from build123d import *

# Parameters (mm, degrees)
F2_W     = 10
F2_H     = 4.472136
F3_W     = 10
F3_H     = 4.472136
F4_W     = 10
F4_H     = 4.472136
F8_ANGLE = -5


with BuildPart() as f5:
    # F4 (on offset) → F5 section 0
    with BuildSketch(Plane.XZ.offset(-30)):
        Polygon((-10, 30), (-10, 34.472136), (-13.577709, 27.316718), (-21.422291, 11.627553), (-25, 4.472136), (-25, 0), align=None)
    # F3 (on Front) → F5 section 1
    with BuildSketch(Plane.XZ):
        Polygon((-10, 30), (-10, 34.472136), (-12.398913, 29.674309), (-13.577709, 27.316718), (-21.422291, 11.627553), (-22.601087, 9.269963), (-25, 4.472136), (-25, 0), align=None)
    # F2 (on offset) → F5 section 2
    with BuildSketch(Plane.XZ.offset(30)):
        Polygon((-10, 30), (-10, 34.472136), (-11.284195, 31.903745), (-12.236068, 30), (-22.763932, 8.944272), (-23.715805, 7.040526), (-25, 4.472136), (-25, 0), align=None)
    loft()

    # F2 (on offset) → F6 section 0
    with BuildSketch(Plane.XZ.offset(30)):
        with Locations((-5, 32.236068)):
            Rectangle(F2_W, F2_H)
    # F3 (on Front) → F6 section 1
    with BuildSketch(Plane.XZ):
        with Locations((-5, 32.236068)):
            Rectangle(F3_W, F3_H)
    # F4 (on offset) → F6 section 2
    with BuildSketch(Plane.XZ.offset(-30)):
        with Locations((-5, 32.236068)):
            Rectangle(F4_W, F4_H)
    loft()

    # F2 (on offset) → F7 section 0
    with BuildSketch(Plane.XZ.offset(30)):
        with Locations((-30, 2.236068)):
            Rectangle(F2_W, F2_H)
    # F3 (on Front) → F7 section 1
    with BuildSketch(Plane.XZ):
        with Locations((-30, 2.236068)):
            Rectangle(F3_W, F3_H)
    # F4 (on offset) → F7 section 2
    with BuildSketch(Plane.XZ.offset(-30)):
        with Locations((-30, 2.236068)):
            Rectangle(F4_W, F4_H)
    loft()

    # F2 (on offset) → F8 (revolve)
    with BuildSketch(Plane.XZ.offset(30)):
        Polygon((-10, 30), (-10, 34.472136), (-11.284195, 31.903745), (-12.236068, 30), (-22.763932, 8.944272), (-23.715805, 7.040526), (-25, 4.472136), (-25, 0), align=None)
        with Locations((-5, 32.236068)):
            Rectangle(F2_W, F2_H)
        with Locations((-30, 2.236068)):
            Rectangle(F2_W, F2_H)
    revolve(axis=Axis((-35, -30, 2.236068), (0, 0, 1)), revolution_arc=F8_ANGLE)


solid = f5.part
Could you check a few things on this model? Use its own coordinates, in mm. A direction names the side the tool comes from. Give positions to 0.01 mm unless a question says otherwise; leave off trailing zeros. Order: outer loops, then holes, each group sorted by start corner. A loop starts at its lowest first (then second) coordinate and runs counter-clockwise, first axis right, second up.
1. I need wall thicknesses on L1, parallel to Z at x = -8.5, y = 27.5; L2, parallel to Z at x = -32, y = 4.5; L3, parallel to X at y = -22.5, z = 3. Which ranges of each line are inside material? Lowest first, please.
Answers below:
L1: z = 30 to 34.47
L2: z = 0 to 4.47
L3: x = -35 to -23.5
2. Which directions (+Z, -Z, +X, -X, +Y, -Y) give clear straight access to the entire face, cutting with the end or side of a thin tool? Please do faces 1 (the flat face through (-5, -2, 30)), 2 (the flat face through (-30, -1, 0)), 3 (the flat face through (-30, -1, 4.472)).
Answers below:
face 1: -Z, +X, +Y, -Y
face 2: -Z, +X, -X, +Y, -Y
face 3: +Z, -X, +Y, -Y
3. Suppose I cut it at B-B (x = -5.5). Write out the boundary of the cut face in (y, z).
Answers below:
outline: (-32.58, 30) - (30, 30) - (30, 34.47) - (-32.58, 34.47) - close
4. For pin 1 (5 mm diameter, centred on x = -23, y = 20.5, fed in from +Z); pin 2 (8 mm diameter, centred on x = -17, y = -4.5, fed in from -Z); pin 3 (1 mm diameter, centred on x = -24, z = 11.5, fed in from -Y); pin 4 (1 mm diameter, centred on y = 21, z = 13, fed in from +X), each with a flat end and sliding along its axis, tell me the tip position at first contact or that it passes through.
Answers below:
pin 1: stops at z = 13.47
pin 2: stops at z = 8
pin 3: passes through
pin 4: stops at x = -18.25
5. Suppose I cut it at A-A (x = -30.5). Write out the boundary of the cut face in (y, z), plus the area to 3 significant figures.
Answers below:
outline: (-30.39, 0) - (30, 0) - (30, 4.47) - (-30.39, 4.47) - close
area: 270 mm2
